Model file for the job. Use its own axes, mm. Face numbers are marked on the shaded views. A direction names the side the tool comes from. Round coordinates to 2 decimals unless told otherwise and drop trailing zeros. Loops run counter-clockwise (first coordinate to the right, second up) from the corner with the lowest first, then second, coordinate; pieces in that order, holes last. Notation, with made-up numbers: M 30.5,58.5 L 77.5,58.5 A15 ccw 77.5,67.5 Z; hole C -27,-14.5 d10. An arc over 180 degrees is marked long. Use a Markdown table: item, result. Add a question column.
Item 1: Tool access for the marked faces 1 and 2: list every direction of +Z, -Z, +X, -X, +Y, -Y with a clear straight run to the whole face (end or side of a thin tool).
Item 2: Saw through at B-B on x = 0. Write the cut outline in (y, z), then the cut area to 3 significant figures.
Item 3: Saw through at D-D on z = 4.75. Write the cut outline in (x, y), then the cut area to 3 significant figures.
Item 4: Wall check: L1, parallel to Y at x = 0, z = 14; L2, parallel to Y at x = 0, z = 16.05; L3, parallel to Y at x = 3.25, z = 12.5. Give the ranges that are in metal, low to high. Write a range as from..to.
Item 5: Pin check, flat tips, straight feed: P1, Ø3, axis at y = -6.5, z = 17, coming from the -X side; P2, Ø4, axis at y = 2.5, z = 6.5, coming from the -X side; P3, Ø8, axis at y = -8.5, z = 8, coming from the -X side. Stop position of each tip, or through.
Item 6: Saw through at A-A on z = 14.25. Write the cut outline in (x, y).
```python
from build123d import *

# Parameters (mm, degrees)
F2_SIZE = 3


with BuildPart() as f1:
    # F0 (on Front) → F1 (revolve)
    with BuildSketch(Plane.XZ):
        Polygon((13.5, 20), (0, 20), (0, 18), (1.5, 18), (1.5, 13), (3, 13), (3, 18), (12.5, 18), (12.5, 0.142242), (13.5, 0), align=None)
    revolve(axis=Axis((0, 0, 25.805777), (0, 0, 1)))

    # F2
    f2_edges = [f1.edges().sort_by_distance(p)[0] for p in [
        (-3, 0, 18),
        (-12.5, 0, 18),
    ]]
    chamfer(f2_edges, length=F2_SIZE)


solid = f1.part
```
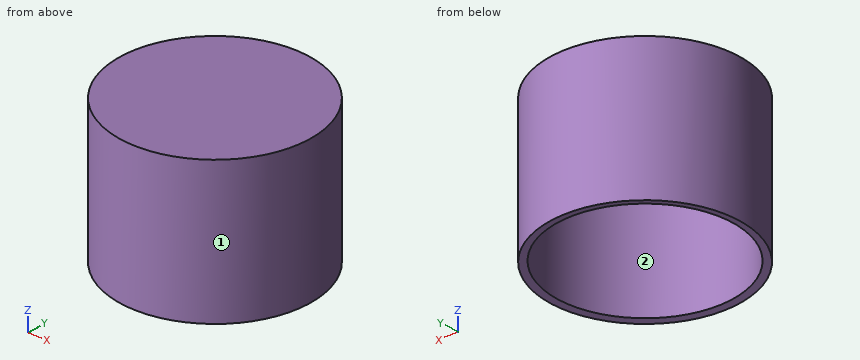
Entries:
| question | item | result |
|---|---|---|
| 1 | face 1 | +Z, -Z |
| 1 | face 2 | -Z |
| 2 | outline | M -13.5,0 L -12.5,0.14 L -12.5,15 L -9.5,18 L -6,18 L -3,15 L -3,13 L -1.5,13 L -1.5,18 L 1.5,18 L 1.5,13 L 3,13 L 3,15 L 6,18 L 9.5,18 L 12.5,15 L 12.5,0.14 L 13.5,0 L 13.5,20 L -13.5,20 Z |
| 2 | area | 123 mm2 |
| 3 | outline | C 0,0 d27; hole C 0,0 d25 |
| 3 | area | 81.7 mm2 |
| 4 | L1 | -13.5..-12.5, -3..-1.5, 1.5..3, 12.5..13.5 |
| 4 | L2 | -13.5..-11.45, -4.05..-1.5, 1.5..4.05, 11.45..13.5 |
| 4 | L3 | -13.1..-12.07, 12.07..13.1 |
| 5 | P1 | x = -12.54 |
| 5 | P2 | x = -13.49 |
| 5 | P3 | x = -12.73 |
| 6 | outline | C 0,0 d27; C 0,0 d6; hole C 0,0 d25; hole C 0,0 d3 |
